from build123d import *

# Parameters (mm, degrees)
SKETCH1_W           = 9.7
SKETCH1_H           = 13
BOSS_EXTRUDE1_DEPTH = 8.5
SKETCH2_R           = 4.5
BOSS_EXTRUDE2_DEPTH = 5
BOSS_EXTRUDE4_START = -5
SKETCH3_R           = 3
BOSS_EXTRUDE4_DEPTH = 21.5
CUT_EXTRUDE1_DEPTH  = 5
CUT_EXTRUDE2_DEPTH  = 12
CHAMFER1_SIZE       = 1
CHAMFER1_SIZE2      = 1.732050808


with BuildPart() as part:
    # Sketch1 → Boss-Extrude1 (new body)
    with BuildSketch(Plane(origin=(0, 0, 0), x_dir=(1, 0, 0), z_dir=(0, 1, 0))):
        Rectangle(SKETCH1_W, SKETCH1_H)
    extrude(amount=BOSS_EXTRUDE1_DEPTH)

    # Sketch2 → Boss-Extrude2 (add)
    with BuildSketch(Plane(origin=(0, 8.5, 0), x_dir=(1, 0, 0), z_dir=(0, 1, 0))):
        Circle(SKETCH2_R)
    extrude(amount=BOSS_EXTRUDE2_DEPTH)

    # Sketch3 → Boss-Extrude4 (add)
    with BuildSketch(Plane(origin=(0, 13.5, 0), x_dir=(1, 0, 0), z_dir=(0, 1, 0)).offset(BOSS_EXTRUDE4_START)):
        Circle(SKETCH3_R)
    extrude(amount=BOSS_EXTRUDE4_DEPTH)

    # Sketch4 → Cut-Extrude1 (cut)
    with BuildSketch(Plane(origin=(0, 13.5, 0), x_dir=(1, 0, 0), z_dir=(0, 1, 0))):
        with BuildLine():
            ThreePointArc((-4, 2.061552813), (-4.5, 0), (-4, -2.061552813))
            Line((-4, -2.061552813), (-4, 2.061552813))
        make_face()
        with BuildLine():
            ThreePointArc((-2.061552813, -4), (0, -4.5), (2.061552813, -4))
            Line((2.061552813, -4), (-2.061552813, -4))
        make_face()
        with BuildLine():
            Line((4, 2.061552813), (4, -2.061552813))
            ThreePointArc((4, -2.061552813), (4.373213921, -1.060660172), (4.5, 0))
            ThreePointArc((4.5, 0), (4.373213921, 1.060660172), (4, 2.061552813))
        make_face()
        with BuildLine():
            Line((-2.061552813, 4), (2.061552813, 4))
            ThreePointArc((2.061552813, 4), (0, 4.5), (-2.061552813, 4))
        make_face()
    extrude(amount=-CUT_EXTRUDE1_DEPTH, mode=Mode.SUBTRACT)

    # Sketch5 → Cut-Extrude2 (cut)
    with BuildSketch(Plane(origin=(0, 30, 0), x_dir=(1, 0, 0), z_dir=(0, 1, 0))):
        with BuildLine():
            Line((0, -3), (-2.598076211, 1.5))
            ThreePointArc((-2.598076211, 1.5), (-2.598076211, -1.5), (0, -3))
        make_face()
    extrude(amount=-CUT_EXTRUDE2_DEPTH, mode=Mode.SUBTRACT)

    # Chamfer1
    chamfer1_edges = [part.edges().sort_by_distance(p)[0] for p in [
        (0.776457135, 30, -2.897777479),
        (-1.299038106, 30, 0.75),
    ]]
    chamfer1_side = [part.faces().sort_by_distance(p)[0] for p in [
        (0.445120094, 30, -0.256990206),
    ]]
    chamfer(chamfer1_edges, length=CHAMFER1_SIZE, length2=CHAMFER1_SIZE2, reference=chamfer1_side[0])


solid = part.part
Part model, mm, in its own coordinate system. A direction names the side the tool comes from. Coordinates: 2 decimals unless noted, no trailing zeros. Order: outer loops, then holes, each group sorted by start corner. A loop starts at its lowest first (then second) coordinate and runs counter-clockwise, first axis right, second up.
(1) Probe L1, parallel to Y at x = -3.5, z = -1.25; L2, parallel to Y at x = 1.5, z = -4.25; L3, parallel to Z at x = 2.75, y = 17.5. List the from-to ranges inside material, lowest first.
Check sheet entries:
L1: y = 0 to 13.5
L2: y = 0 to 8.5
L3: z = -1.2 to 1.2
(2) Slice it at D-D, the plane y = 22. Write the cut outline in (x, z).
Check sheet entries:
outline: (-2.6, -1.5) arc R3 ccw (long way) to (0, 3) - close
(3) Slice it at A-A, the plane y = 17.5. Write the cut outline in (x, z).
Check sheet entries:
outline: circle Ø6 at (0, 0)
(4) Slice it at C-C, the plane z = 5.5. Write the cut outline in (x, y), and give its area (4 significant figures).
Check sheet entries:
outline: (-4.85, 0) - (4.85, 0) - (4.85, 8.5) - (-4.85, 8.5) - close
area: 82.45 mm2
(5) Tool access for faces 1 (the face through (3, 13.5, 2)), 2 (the face through (3.196, 10.965, -3.168)), 3 (the face through (3.168, 10.965, 3.196)), 4 (the face through (-1.28, 23.21, 0.78)): list every direction of +Z, -Z, +X, -X, +Y, -Y with a clear straight run to the whole face (end or side of a thin tool).
Check sheet entries:
face 1: +Y
face 2: -Z, +X, +Y
face 3: +Z, +X, +Y
face 4: +Z, -X, +Y
(6) Slice it at B-B, the plane z = 0. Write the cut outline in (x, y), and give its area (3 significant figures).
Check sheet entries:
outline: (-4.85, 0) - (4.85, 0) - (4.85, 8.5) - (4, 8.5) - (4, 13.5) - (3, 13.5) - (3, 28.27) - (2, 30) - (-0.58, 30) - (-1.73, 28.27) - (-1.73, 18) - (-3, 18) - (-3, 13.5) - (-4, 13.5) - (-4, 8.5) - (-4.85, 8.5) - close
area: 204 mm2
(7) Pin check, flat tips, straight feed: pin 1 Ø1.5 at (y, z) = (10, -1) entering from -X; pin 2 Ø4.5 at (x, y) = (1, 12) entering from +Z; pin 3 Ø6 at (y, z) = (17.5, 3.5) entering from +X. Stop position of each tip, or through.
Check sheet entries:
pin 1: stops at x = -4
pin 2: stops at z = 4
pin 3: stops at x = 2.96
